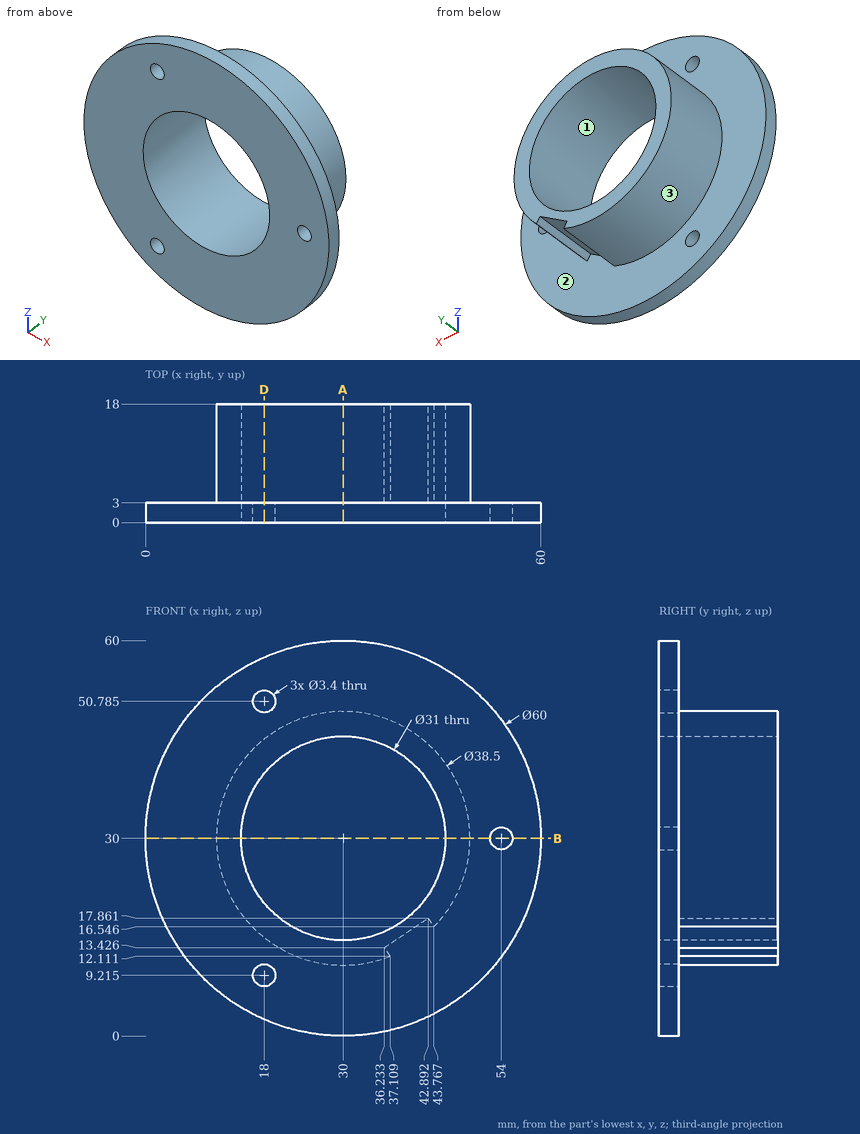
Input: dimensioned drawing with shaded views. Units: mm. Origin: part minimum x, y, z. Coordinates: 2 decimals unless noted, no trailing zeros. Loops run counter-clockwise (first coordinate to the right, second up) from the corner with the lowest first, then second, coordinate; pieces in that order, holes last. Notation, with made-up numbers: (-8.5, -26) -> (21.5, -26) arc R33 cw to (21.5, 6) -> close; hole circle Ø5 at (38, 22). An arc over 180 degrees is marked (long way). Use a Markdown table: item, result. Add a question column.
(1) Section query A-A, the plane x = 30. Return loops of the section in (y, z).
(2) Line query: line 1 along X through (y, z) = (1.65, 30); line 2 along X through (y, z) = (14.25, 30); line 3 along Y through (x, z) = (6.5, 32). Output: solid intervals per line, ascending.
(3) Section query B-B, the plane z = 30. Return loops of the section in (x, y).
(4) Section query D-D, the plane x = 18. Return loops of the section in (y, z) (1 decimal).
(5) Mould query, pull axis Z, two halves, no side actions, for the marked faces 1, 2 and 3. Classes: pulls with the +Z half, pulls with the -Z half, needs draft (parallel to the pull), parting line crosses it, or undercut.
(6) Pin query (flat end, axial travel): pin 1 Ø10 at (y, z) = (11, 28.5) entering from -X; pin 2 Ø5.5 at (x, z) = (54, 30) entering from +Y; pin 3 Ø10 at (y, z) = (12, 12.5) entering from +X. Return the tip coordinate at first contact, or that it passes through.
Answer:
| question | item | result |
|---|---|---|
| 1 | outline | (0, 0) -> (3, 0) -> (3, 10.75) -> (18, 10.75) -> (18, 14.5) -> (0, 14.5) -> close; (0, 45.5) -> (18, 45.5) -> (18, 49.25) -> (3, 49.25) -> (3, 60) -> (0, 60) -> close |
| 2 | line 1 | x = 0 to 14.5, 45.5 to 52.3, 55.7 to 60 |
| 2 | line 2 | x = 10.75 to 14.5, 45.5 to 49.25 |
| 2 | line 3 | y = 0 to 3 |
| 3 | outline | (0, 0) -> (14.5, 0) -> (14.5, 18) -> (10.75, 18) -> (10.75, 3) -> (0, 3) -> close; (45.5, 0) -> (52.3, 0) -> (52.3, 3) -> (49.25, 3) -> (49.25, 18) -> (45.5, 18) -> close; (55.7, 0) -> (60, 0) -> (60, 3) -> (55.7, 3) -> close |
| 4 | outline | (0, 2.5) -> (3, 2.5) -> (3, 7.5) -> (0, 7.5) -> close; (0, 10.9) -> (3, 10.9) -> (3, 14.9) -> (18, 14.9) -> (18, 20.2) -> (0, 20.2) -> close; (0, 39.8) -> (18, 39.8) -> (18, 45.1) -> (3, 45.1) -> (3, 49.1) -> (0, 49.1) -> close; (0, 52.5) -> (3, 52.5) -> (3, 57.5) -> (0, 57.5) -> close |
| 5 | face 1 | undercut |
| 5 | face 2 | needs draft |
| 5 | face 3 | parting line crosses it |
| 6 | pin 1 | stops at x = 10.75 |
| 6 | pin 2 | stops at y = 3 |
| 6 | pin 3 | stops at x = 44.64 |
